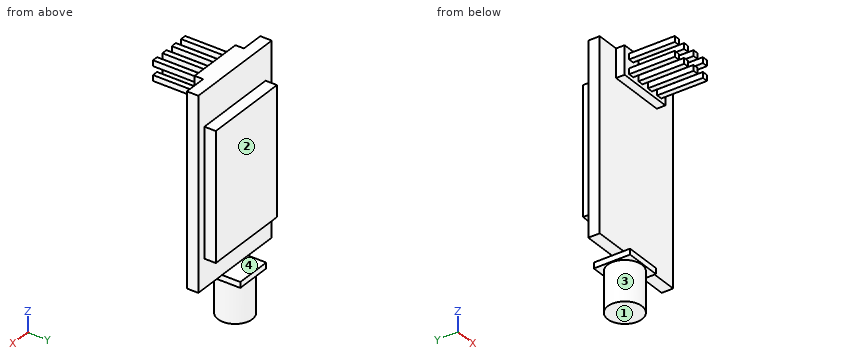
Autodesk Inventor part; units mm, degrees
ref_plane "YZ Plane" through (0, 0, 0) normal (1, 0, 0) x (0, 1, 0)
ref_plane "XZ Plane" through (0, 0, 0) normal (0, 1, 0) x (-1, 0, 0)
ref_plane "XY Plane" through (0, 0, 0) normal (0, 0, 1) x (1, 0, 0)
sketch "Sketch1" plane through (0, 0, 0) normal (0, 1, 0) x (-1, 0, 0)
  line L0 (0, 0) -> (18, 0)
  line L1 (18, 0) -> (18, -33.3)
  line L2 (18, -33.3) -> (0, -33.3)
  line L3 (0, -33.3) -> (0, 0)
  dimension "d0" = 33.3
  dimension "d1" = 18
extrude "Extrusion1" add sketch "Sketch1" along normal blind 2
sketch "Sketch2" plane through (0, 2, 0) normal (0, 1, 0) x (1, 0, 0)
  line L0 (-16.5, 6) -> (-1.5, 6)
  line L1 (-1.5, 6) -> (-1.5, 28.3)
  line L2 (-1.5, 28.3) -> (-16.5, 28.3)
  line L3 (-16.5, 28.3) -> (-16.5, 6)
  line L4 (-18, 0) -> (0, 0)
  line L5 (0, 33.3) -> (-18, 33.3)
  line L6 (-18, 33.3) -> (-18, 0)
  line L7 (0, 0) -> (0, 33.3)
  dimension "d4" = 6
  dimension "d5" = 5
  dimension "d6" = 1.5
  dimension "d7" = 1.5
extrude "Extrusion2" add sketch "Sketch2" along normal blind 2 contours L3 L2 L1 L0
sketch "Sketch3" plane through (0, 0, -33.3) normal (0, 0, -1) x (-1, 0, 0)
  line L0 (18, 0) -> (0, 0) construction
  line L1 (18, 0) -> (18, 2) construction
  line L2 (0, 2) -> (18, 2) construction
  line L3 (0, 0) -> (0, 2) construction
  line L4 (5.825, 5.2) -> (12.175, 5.2)
  line L5 (12.175, 5.2) -> (12.175, -1.15)
  line L6 (12.175, -1.15) -> (5.825, -1.15)
  line L7 (5.825, -1.15) -> (5.825, 5.2)
  point P0 (0, 0)
  point P1 (9, 5.2)
  point P2 (9, 2)
  dimension "d10" = 6.35
  dimension "d11" = 6.35
  dimension "d12" = 3.2
extrude "Extrusion3" add sketch "Sketch3" along normal blind 1
sketch "Sketch4" plane through (0, 0, -34.3) normal (0, 0, -1) x (-1, 0, 0)
  line L0 (12.175, 5.2) -> (5.825, 5.2) construction
  line L1 (5.825, 5.2) -> (5.825, -1.15) construction
  line L2 (5.825, -1.15) -> (12.175, -1.15) construction
  line L3 (12.175, -1.15) -> (12.175, 5.2) construction
  circle A0 centre (9, 2.025) radius 3
  point P0 (0, 0)
  dimension "d15" = 6
extrude "Extrusion4" add sketch "Sketch4" along normal blind 7
sketch "Sketch5" plane through (0, 0, 0) normal (0, -1, 0) x (1, 0, 0)
  line L0 (-18, 0) -> (0, 0)
  line L1 (-4, 0) -> (-14, 0)
  line L2 (-14, 0) -> (-14, -5)
  line L3 (-14, -5) -> (-4, -5)
  line L4 (-4, -5) -> (-4, 0)
  point P0 (-9, -5)
  point P1 (-9, 0)
  dimension "d18" = 5
  dimension "d19" = 10
extrude "Extrusion5" add sketch "Sketch5" along normal blind 1.5
sketch "Sketch6" plane through (0, -1.5, 0) normal (0, -1, 0) x (1, 0, 0)
  line L0 (-6, -1.8409) -> (-5, -1.8409)
  line L1 (-5, -1.8409) -> (-5, -0.8409)
  line L2 (-5, -0.8409) -> (-6, -0.8409)
  line L3 (-6, -0.8409) -> (-6, -1.8409)
  line L4 (-6, -4.3409) -> (-5, -4.3409)
  line L5 (-5, -4.3409) -> (-5, -3.3409)
  line L6 (-5, -3.3409) -> (-6, -3.3409)
  line L7 (-6, -3.3409) -> (-6, -4.3409)
  line L8 (-4, -5) -> (-4, 0)
  point P0 (0, 0)
  dimension "d22" = 1
  dimension "d23" = 1
  dimension "d24" = 1
  dimension "d25" = 1.5
  dimension "d26" = 1
extrude "Extrusion6" add sketch "Sketch6" along normal blind 8
pattern_linear "Rectangular Pattern1" count 4 spacing 2.3 along (-1, 0, 0) of "Extrusion6"
properties part number "SPIRadio" material "ABS Plastic"
Could you check a few things on this model? Use its own coordinates, in mm. Face numbers are marked on the shaded views. A direction names the side the tool comes from. Give positions to 0.01 mm unless a question says otherwise; leave off trailing zeros. Order: outer loops, then holes, each group sorted by start corner. A loop starts at its lowest first (then second) coordinate and runs counter-clockwise, first axis right, second up.
Q1. I'm going to push flat-ended pins straight in: P1, Ø0.6, axis at x = -2.5, y = 1, coming from the -Z side; P2, Ø1.5, axis at x = -5.5, y = -7, coming from the +Z side; P3, Ø1.5, axis at y = 2.5, z = -36.5, coming from the +X side. Where does each tip first touch, or does it pass through?
Q2. Suppose I cut it at B-B, the plane y = -0.5. Write out the boundary of the cut face in (x, z) (3 decimals), and give its area (3 significant figures).
Q3. For the marked faces 1, 2, 3 and 4, which set-ups out of +Z, -Z, +X, -X, +Y, -Y let a thin tool reach every point of the face, with its end or its side?
Q4. Suppose I cut it at A-A, the plane y = -8. Count the separate pieces of the cut face and the enclosed holes in it, and give its area (3 significant figures).
Q5. Suppose I cut it at C-C, the plane z = -16. Write out the boundary of the cut face in (x, y).
Q6. If I drill on line 1 along Z through (x, y) = (-12, -3.25); line 2 along Z through (x, y) = (-8.5, -0.5); line 3 along Y through (x, z) = (-15.5, -24.5), over which ranges is the centre line in solid material (lowest first)?
Q7. Suppose I cut it at D-D, the plane x = -9. Write out the boundary of the cut face in (y, z) (3 decimals).
Solution:
1. P1: stops at z = -33.3
1. P2: stops at z = -0.84
1. P3: stops at x = -6
2. outline: (-14, -5) - (-4, -5) - (-4, 0) - (-14, 0) - close; (-12.175, -34.3) - (-10.62, -34.3) - (-10.62, -41.3) - (-7.38, -41.3) - (-7.38, -34.3) - (-5.825, -34.3) - (-5.825, -33.3) - (-12.175, -33.3) - close
2. area: 79.0 mm2
3. face 1: -Z, +X, -X, +Y, -Y
3. face 2: +Z, +X, -X, +Y
3. face 3: -Z
3. face 4: +X, -X, +Y
4. separate pieces: 8
4. enclosed holes: 0
4. area: 8.00 mm2
5. outline: (-18, 0) - (0, 0) - (0, 2) - (-1.5, 2) - (-1.5, 4) - (-16.5, 4) - (-16.5, 2) - (-18, 2) - close
6. line 1: z = -4.34 to -3.34, -1.84 to -0.84
6. line 2: z = -41.3 to -33.3, -5 to 0
6. line 3: y = 0 to 4
7. outline: (-1.5, -5) - (0, -5) - (0, -33.3) - (-1.15, -33.3) - (-1.15, -34.3) - (-0.975, -34.3) - (-0.975, -41.3) - (5.025, -41.3) - (5.025, -34.3) - (5.2, -34.3) - (5.2, -33.3) - (2, -33.3) - (2, -28.3) - (4, -28.3) - (4, -6) - (2, -6) - (2, 0) - (-1.5, 0) - close
